Part model, mm, in its own coordinate system. Face numbers are marked on the shaded views. A direction names the side the tool comes from. Coordinates: 2 decimals unless noted, no trailing zeros. Order: outer loops, then holes, each group sorted by start corner. A loop starts at its lowest first (then second) coordinate and runs counter-clockwise, first axis right, second up. Notation, with made-up numbers: (-21.5, 25.5) - (-6.5, 25.5) arc R16 ccw to (-6.5, 33.5) - close; hole circle Ø4 at (-17.5, 10.5). An arc over 180 degrees is marked (long way). Use a Markdown table: item, result. Add a question column.
1) Tool access for the marked faces 1, 2 and 3: list every direction of +Z, -Z, +X, -X, +Y, -Y with a clear straight run to the whole face (end or side of a thin tool).
2) Drop flat-ended pins along their axis: P1, Ø0.5, axis at x = -20, y = 6.5, coming from the -Z side; P2, Ø10, axis at y = -7.5, z = 2, coming from the +X side; P3, Ø3, axis at x = 0, z = 6, coming from the +Y side; P4, Ø4, axis at y = 22.5, z = 11.5, coming from the +X side. Give the stop position or say it passes through.
3) Saw through at A-A on z = 6. List the corners of the cut face in (x, y) (3 decimals), then the cut area to 3 significant figures.
4) Saw through at B-B on z = -1.25. List the corners of the cut face in (x, y), then the cut area to 3 significant figures.
5) Saw through at C-C on y = 29. List the corners of the cut face in (x, z) (3 decimals), then the cut area to 3 significant figures.
6) Wall check: L1, parallel to Y at x = 0, z = -0.25; L2, parallel to X at y = 23.75, z = 6 (3 decimals); L3, parallel to X at y = 14, z = 7.5. Give the ranges that are in metal, low to high. Write a range as [from, to].
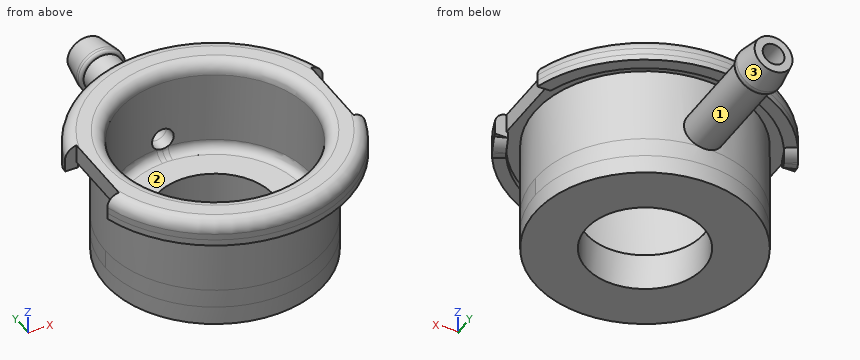
```python
from build123d import *

# Parameters (mm, degrees)
SKETCH1_R                = 17.65
SKETCH1_R_2              = 15.5
BOSS_EXTRUDE1_DEPTH      = 18
BOSS_EXTRUDE2_START      = -3
SKETCH2_R                = 21.65
SKETCH2_R_2              = 15.5
BOSS_EXTRUDE2_DEPTH      = 3
SKETCH3_W                = 5
SKETCH3_H                = 12.5
CUT_EXTRUDE1_DEPTH       = 36.516826998
BOSS_EXTRUDE3_START      = 1
BOSS_EXTRUDE3_DEPTH      = 1
BOSS_EXTRUDE4_START      = 1
BOSS_EXTRUDE4_DEPTH      = 1
CIRPATTERN1_COUNT        = 2
FILLET1_R                = 3
FILLET2_R                = 2
SKETCH6_R                = 1.75
CUT_EXTRUDE2_DEPTH       = 35.96258732
BOSS_EXTRUDE5_REACH      = 74.963
BOSS_EXTRUDE5_END_RADIUS = 17.65
BOSS_EXTRUDE5_START      = 38
SKETCH6_4_R              = 3.175
SKETCH6_4_R_2            = 1.75
SKETCH7_R                = 3.755
SKETCH7_R_2              = 1.75
BOSS_EXTRUDE6_DEPTH      = 5
CHAMFER1_SIZE            = 4
CHAMFER1_SIZE2           = 0.705307923
BOSS_EXTRUDE7_DEPTH      = 3
BOSS_EXTRUDE7_DEPTH_BACK = 3
SKETCH8_R                = 17.65
SKETCH8_R_2              = 9.5
FILLET4_R                = 1.5
FILLET5_R                = 0.5


with BuildPart() as part:
    # Sketch1 → Boss-Extrude1 (new body)
    with BuildSketch(Plane.XY):
        Circle(SKETCH1_R)
        Circle(SKETCH1_R_2, mode=Mode.SUBTRACT)
    extrude(amount=BOSS_EXTRUDE1_DEPTH)

    # Sketch2 → Boss-Extrude2 (add)
    with BuildSketch(Plane.XY.offset(18).offset(BOSS_EXTRUDE2_START)):
        Circle(SKETCH2_R)
        Circle(SKETCH2_R_2, mode=Mode.SUBTRACT)
    extrude(amount=BOSS_EXTRUDE2_DEPTH)

    # Sketch3 → Cut-Extrude1 (cut, through all)
    with BuildSketch(Plane.XY.offset(18)):
        with Locations((21.38, 0)):
            Rectangle(SKETCH3_W, SKETCH3_H)
        with Locations((-21.38, 0)):
            Rectangle(SKETCH3_W, SKETCH3_H)
    extrude(amount=-CUT_EXTRUDE1_DEPTH, mode=Mode.SUBTRACT)

    # Sketch4 → Boss-Extrude3 (add)
    with BuildSketch(Plane(origin=(0, 0, 15), x_dir=(-1, 0, 0), z_dir=(0, 0, -1)).offset(BOSS_EXTRUDE3_START)):
        with BuildLine():
            Line((-20.728241604, -6.25), (-18.629546425, -6.25))
            ThreePointArc((-18.629546425, -6.25), (0, -19.65), (18.629546425, -6.25))
            Line((18.629546425, -6.25), (20.728241604, -6.25))
            ThreePointArc((20.728241604, -6.25), (0, -21.65), (-20.728241604, -6.25))
        make_face()
        with BuildLine():
            Line((-20.728241604, 6.25), (-18.629546425, 6.25))
            ThreePointArc((-18.629546425, 6.25), (0, 19.65), (18.629546425, 6.25))
            Line((18.629546425, 6.25), (20.728241604, 6.25))
            ThreePointArc((20.728241604, 6.25), (0, 21.65), (-20.728241604, 6.25))
        make_face()
    extrude(amount=-BOSS_EXTRUDE3_DEPTH)

    # Sketch5 → Boss-Extrude4 (add)
    with BuildSketch(Plane(origin=(0, 0, 14), x_dir=(-1, 0, 0), z_dir=(0, 0, -1)).offset(BOSS_EXTRUDE4_START)):
        with BuildLine():
            Line((-18.629546425, -6.25), (-20.525683466, -6.886132316))
            ThreePointArc((-20.525683466, -6.886132316), (-19.593212906, -9.210239302), (-18.398607414, -11.411123749))
            Line((-18.398607414, -11.411123749), (-16.698967007, -10.356978368))
            ThreePointArc((-16.698967007, -10.356978368), (-17.783216333, -8.359408882), (-18.629546425, -6.25))
        make_face()
    boss_extrude4 = extrude(amount=-BOSS_EXTRUDE4_DEPTH)

    # CirPattern1: Boss-Extrude4 ×2 about axis
    cirpattern1_axis = Axis((0, 0, 0), (0, 0, 1))
    for i in range(1, CIRPATTERN1_COUNT):
        add(boss_extrude4.rotate(cirpattern1_axis, i * 360 / CIRPATTERN1_COUNT))

    # Fillet1
    # the kernel refuses this fillet: 3 mm, written as the material it takes off along each edge
    with BuildSketch(Plane(origin=(-23.149246776, 14.357549661, 13), x_dir=(0, 0, 1), z_dir=(0.8498202038966606, -0.527072690479253, 0))) as fillet1_piece_1_section:
        with BuildLine():
            CenterArc((3, 2.236067977), FILLET1_R, 180, 48.189685104)
            Line((0, 2.236067977), (0, 0))
            Line((0, 0), (1, 0))
        make_face()
    fillet1_piece_1 = extrude(amount=13.180339887, mode=Mode.PRIVATE)
    fillet1_piece_1 = fillet1_piece_1 - Plane(origin=(0, 0, 13.255909987), x_dir=(0.9480685203545537, 0.3180661577608143, 0), z_dir=(0, 0, -1)) * Cylinder(19.65, 36, mode=Mode.PRIVATE)
    add(fillet1_piece_1, mode=Mode.SUBTRACT)
    with BuildSketch(Plane(origin=(-13.329682278, 4.471956125, 13), x_dir=(0, 0, 1), z_dir=(-0.9480685203545541, 0.3180661577608135, 0))) as fillet1_piece_2_section:
        with BuildLine():
            CenterArc((3, 2.236067977), FILLET1_R, 180, 48.189685104)
            Line((0, 2.236067977), (0, 0))
            Line((0, 0), (1, 0))
        make_face()
    fillet1_piece_2 = extrude(amount=13.180339887, mode=Mode.PRIVATE)
    fillet1_piece_2 = fillet1_piece_2 - Plane(origin=(0, 0, 13.255909987), x_dir=(0.9480685203545537, 0.3180661577608143, 0), z_dir=(0, 0, -1)) * Cylinder(19.65, 36, mode=Mode.PRIVATE)
    add(fillet1_piece_2, mode=Mode.SUBTRACT)
    with BuildSketch(Plane(origin=(23.149246776, -14.357549661, 13), x_dir=(0, 0, 1), z_dir=(-0.8498202038966607, 0.5270726904792529, 0))) as fillet1_piece_3_section:
        with BuildLine():
            CenterArc((3, 2.236067977), FILLET1_R, 180, 48.189685104)
            Line((0, 2.236067977), (0, 0))
            Line((0, 0), (1, 0))
        make_face()
    fillet1_piece_3 = extrude(amount=13.180339887, mode=Mode.PRIVATE)
    fillet1_piece_3 = fillet1_piece_3 - Plane(origin=(0, 0, 13.255909987), x_dir=(0.9480685203545538, -0.3180661577608143, 0), z_dir=(0, 0, -1)) * Cylinder(19.65, 36, mode=Mode.PRIVATE)
    add(fillet1_piece_3, mode=Mode.SUBTRACT)
    with BuildSketch(Plane(origin=(13.329682278, -4.471956125, 13), x_dir=(-0.3180661577608133, -0.9480685203545539, 0), z_dir=(0.9480685203545541, -0.3180661577608134, 0))) as fillet1_piece_4_section:
        with BuildLine():
            CenterArc((2.236067977, -3), FILLET1_R, 90, 48.189685104)
            Line((0, -1), (0, 0))
            Line((0, 0), (2.236067977, 0))
        make_face()
    fillet1_piece_4 = extrude(amount=13.180339887, mode=Mode.PRIVATE)
    fillet1_piece_4 = fillet1_piece_4 - Plane(origin=(0, 0, 13.255909987), x_dir=(0.9480685203545538, -0.3180661577608143, 0), z_dir=(0, 0, -1)) * Cylinder(19.65, 36, mode=Mode.PRIVATE)
    add(fillet1_piece_4, mode=Mode.SUBTRACT)

    # Fillet2
    fillet2_edges = [part.edges().sort_by_distance(p)[0] for p in [
        (0, 21.65, 18),
        (-15.5, 0, 18),
        (0, -21.65, 18),
    ]]
    fillet(fillet2_edges, radius=FILLET2_R)

    # Sketch6 → Cut-Extrude2 (cut, through all)
    with BuildSketch(Plane(origin=(0, 0, 0), x_dir=(1, 0, 0), z_dir=(0, 1, 0))):
        with Locations(Location((0, -6, 0), (0, 0, 90))):
            Circle(SKETCH6_R)
    extrude(amount=CUT_EXTRUDE2_DEPTH, mode=Mode.SUBTRACT)

    # Boss-Extrude5: up to this cylinder (the profile starts outside it)
    boss_extrude5_end = Plane(origin=(0, 0, 2.914803), z_dir=(0, 0, -1)) * Cylinder(BOSS_EXTRUDE5_END_RADIUS, 186.226, mode=Mode.PRIVATE)
    # Sketch6<4> → Boss-Extrude5 (add, up to the surface)
    with BuildSketch(Plane(origin=(0, 0, 0), x_dir=(1, 0, 0), z_dir=(0, 1, 0)).offset(BOSS_EXTRUDE5_START), mode=Mode.PRIVATE) as boss_extrude5_sk1:
        with Locations(Location((0, -6, 0), (0, 0, 270))):
            Circle(SKETCH6_4_R)
        with Locations(Location((0, -6, 0), (0, 0, 90))):
            Circle(SKETCH6_4_R_2, mode=Mode.SUBTRACT)
    boss_extrude5_tool1 = extrude(boss_extrude5_sk1.sketch, amount=-BOSS_EXTRUDE5_REACH, mode=Mode.PRIVATE) - boss_extrude5_end
    add(boss_extrude5_tool1.solids().sort_by_distance((0, 38, 2.914803))[0])

    # Sketch7 → Boss-Extrude6 (add)
    with BuildSketch(Plane(origin=(0, 38, 0), x_dir=(1, 0, 0), z_dir=(0, 1, 0))):
        with Locations(Location((0, -6, 0), (0, 0, 270))):
            Circle(SKETCH7_R)
        with Locations(Location((0, -6, 0), (0, 0, 90))):
            Circle(SKETCH7_R_2, mode=Mode.SUBTRACT)
    extrude(amount=-BOSS_EXTRUDE6_DEPTH)

    # Chamfer1
    chamfer1_edges = [part.edges().sort_by_distance(p)[0] for p in [
        (0, 38, 2.245),
    ]]
    chamfer1_side = [part.faces().sort_by_distance(p)[0] for p in [
        (0, 35.5, 2.245),
    ]]
    chamfer(chamfer1_edges, length=CHAMFER1_SIZE, length2=CHAMFER1_SIZE2, reference=chamfer1_side[0])

    # Sketch8 → Boss-Extrude7 (add, two sides: drawn at the far end of the back side and taken through both)
    with BuildSketch(Plane(origin=(0, 0, 0), x_dir=(-1, 0, 0), z_dir=(0, 0, -1)).offset(-BOSS_EXTRUDE7_DEPTH_BACK)):
        Circle(SKETCH8_R)
        Circle(SKETCH8_R_2, mode=Mode.SUBTRACT)
    extrude(amount=BOSS_EXTRUDE7_DEPTH + BOSS_EXTRUDE7_DEPTH_BACK)

    # Fillet4
    fillet4_edges = [part.edges().sort_by_distance(p)[0] for p in [
        (-15.5, 0, 3),
    ]]
    fillet(fillet4_edges, radius=FILLET4_R)

    # Fillet5
    fillet5_edges = [part.edges().sort_by_distance(p)[0] for p in [
        (0, 33, 2.245),
    ]]
    fillet(fillet5_edges, radius=FILLET5_R)


solid = part.part
```
Results are:
| question | item | result |
|---|---|---|
| 1 | face 1 | none |
| 1 | face 2 | +Z |
| 1 | face 3 | +Y |
| 2 | P1 | z = 13.94 |
| 2 | P2 | x = 17.47 |
| 2 | P3 | y = -15.43 |
| 2 | P4 | through |
| 3 | outline | (-3.755, 33.5) arc R0.5 ccw to (-3.255, 33) - (-3.175, 33) - (-3.175, 17.362) arc R17.65 ccw (long way) to (3.175, 17.362) - (3.175, 33) - (3.255, 33) arc R0.5 ccw to (3.755, 33.5) - (3.755, 34) - (3.05, 38) - (1.75, 38) - (1.75, 15.401) arc R15.5 cw (long way) to (-1.75, 15.401) - (-1.75, 38) - (-3.05, 38) - (-3.755, 34) - close |
| 3 | area | 278 mm2 |
| 4 | outline | circle Ø35.3 at (0, 0); hole circle Ø19 at (0, 0) |
| 4 | area | 695 mm2 |
| 5 | outline | circle Ø6.35 at (0, 6); hole circle Ø3.5 at (0, 6) |
| 5 | area | 22.0 mm2 |
| 6 | L1 | [-17.65, -9.5], [9.5, 17.65] |
| 6 | L2 | [-3.175, -1.75], [1.75, 3.175] |
| 6 | L3 | [-10.75, -6.65], [6.65, 10.75] |
